from build123d import *

# Parameters (mm, degrees)
PAD005_DEPTH         = 2
POCKET003_DEPTH      = 2
SKETCH009_R          = 2.7
PAD004_DEPTH         = 5.9
SKETCH013_W          = 25
SKETCH013_H          = 50.4
SKETCH013_H_2        = 36.4
POCKET007_DEPTH      = 5.901
POCKET007_DEPTH_BACK = 0.001
SKETCH016_W          = 2.35
SKETCH016_H          = 50.4
PAD008_DEPTH         = 15
SKETCH017_W          = 2.35
SKETCH017_H          = 36.4
PAD009_DEPTH         = 5
SKETCH019_R          = 2.9
POCKET009_DEPTH      = 1.5
PAD011_DEPTH         = 5
SKETCH023_W          = 8
SKETCH023_H          = 4.5
SKETCH023_W_2        = 10
PAD013_DEPTH         = 7
SKETCH025_R          = 1.25
POCKET011_DEPTH      = 17.001
POCKET011_DEPTH_BACK = 0.001
SKETCH033_W          = 20
SKETCH033_H          = 50
POCKET017_DEPTH      = 17.001
POCKET017_DEPTH_BACK = 0.001
SKETCH042_W          = 15
SKETCH042_H          = 5.8
SKETCH042_H_2        = 3
POCKET021_DEPTH      = 17.001
POCKET021_DEPTH_BACK = 0.001


with BuildPart() as part:
    # Sketch011 → Pad005 (new body)
    with BuildSketch(Plane.XY):
        with BuildLine():
            Line((-29.5, -64), (29.5, -64))
            ThreePointArc((29.5, -64), (31.267767, -63.267767), (32, -61.5))
            Line((32, -42.5), (32, -61.5))
            ThreePointArc((34.5, -40), (32.732233, -40.732233), (32, -42.5))
            Line((34.5, 12), (34.5, -40))
            ThreePointArc((32, 14.5), (32.732233, 12.732233), (34.5, 12))
            Line((32, 21.5), (32, 14.5))
            ThreePointArc((32, 21.5), (31.267767, 23.267767), (29.5, 24))
            Line((29.5, 24), (-34.5, 24))
            ThreePointArc((-34.5, 24), (-36.267767, 23.267767), (-37, 21.5))
            Line((-37, 21.5), (-37, -40))
            ThreePointArc((-37, -40), (-36.267767, -41.767767), (-34.5, -42.5))
            ThreePointArc((-32, -45), (-32.732233, -43.232233), (-34.5, -42.5))
            Line((-32, -45), (-32, -61.5))
            ThreePointArc((-32, -61.5), (-31.267767, -63.267767), (-29.5, -64))
        make_face()
    extrude(amount=-PAD005_DEPTH)

    # Sketch007 → Pocket003 (cut)
    with BuildSketch(Plane.XY):
        Polygon((-21, 18.3), (-21, 5.3), (21, 5.3), (21, -3.7), (28, -3.7), (28, 18.3), align=None)
    extrude(amount=-POCKET003_DEPTH, mode=Mode.SUBTRACT)

    # Sketch009 → Pad004 (join)
    with BuildSketch(Plane.XY):
        with Locations((-18.25, -26)):
            Circle(SKETCH009_R)
        with Locations((12.75, -21)):
            Circle(SKETCH009_R)
        with Locations((18.25, 2.5027)):
            Circle(SKETCH009_R)
    extrude(amount=-PAD004_DEPTH)

    # Sketch013 → Pocket007 (cut, two sides)
    with BuildSketch(Plane.XY) as pocket007_sk:
        with Locations((-43.3, -8)):
            Rectangle(SKETCH013_W, SKETCH013_H)
        with Locations((43.3, -10)):
            Rectangle(SKETCH013_W, SKETCH013_H_2)
    extrude(amount=-POCKET007_DEPTH, mode=Mode.SUBTRACT)
    extrude(pocket007_sk.sketch, amount=POCKET007_DEPTH_BACK, mode=Mode.SUBTRACT)

    # Sketch016 (on Face5 of Pocket007) → Pad008 (join)
    with BuildSketch(Plane(origin=(0, 0, -2), x_dir=(1, 0, 0), z_dir=(0, 0, -1))):
        with Locations((-29.625, 8)):
            Rectangle(SKETCH016_W, SKETCH016_H)
    extrude(amount=PAD008_DEPTH)

    # Sketch017 (on Face5 of Pocket007) → Pad009 (join)
    with BuildSketch(Plane(origin=(0, 0, -2), x_dir=(1, 0, 0), z_dir=(0, 0, -1))):
        with Locations((29.625, 10)):
            Rectangle(SKETCH017_W, SKETCH017_H)
    extrude(amount=PAD009_DEPTH)

    # Sketch019 → Pocket009 (cut)
    with BuildSketch(Plane.XY):
        with Locations((-15, 21)):
            Circle(SKETCH019_R)
        with Locations((15, 21)):
            Circle(SKETCH019_R)
        with Locations((-15, -55)):
            Circle(SKETCH019_R)
        with Locations((15, -55)):
            Circle(SKETCH019_R)
    extrude(amount=-POCKET009_DEPTH, mode=Mode.SUBTRACT)

    # Sketch021 (on Face5 of Pocket009) → Pad011 (join)
    with BuildSketch(Plane(origin=(0, 0, -2), x_dir=(1, 0, 0), z_dir=(0, 0, -1))):
        with BuildLine():
            Line((-29.5, 64), (29.5, 64))
            ThreePointArc((32, 61.5), (31.267767, 63.267767), (29.5, 64))
            Line((32, 61.5), (32, 42.5))
            ThreePointArc((32, 42.5), (32.732233, 40.732233), (34.5, 40))
            Line((34.5, 28.2), (34.5, 40))
            Line((29, 28.2), (34.5, 28.2))
            Line((29, 58.5), (29, 28.2))
            Line((-29, 58.5), (29, 58.5))
            Line((-29, 39.5), (-29, 58.5))
            Line((-34, 39.5), (-29, 39.5))
            Line((-34, 33.2), (-34, 39.5))
            Line((-37, 33.2), (-34, 33.2))
            Line((-37, 40), (-37, 33.2))
            ThreePointArc((-34.5, 42.5), (-36.267767, 41.767767), (-37, 40))
            ThreePointArc((-34.5, 42.5), (-32.732233, 43.232233), (-32, 45))
            Line((-32, 61.5), (-32, 45))
            ThreePointArc((-29.5, 64), (-31.267767, 63.267767), (-32, 61.5))
        make_face()
        with BuildLine():
            Line((34.5, -8.2), (34.5, -12))
            ThreePointArc((34.5, -12), (32.732233, -12.732233), (32, -14.5))
            Line((32, -14.5), (32, -21.5))
            ThreePointArc((29.5, -24), (31.267767, -23.267767), (32, -21.5))
            Line((29.5, -24), (-34.5, -24))
            ThreePointArc((-37, -21.5), (-36.267767, -23.267767), (-34.5, -24))
            Line((-37, -21.5), (-37, -17.2))
            Line((-37, -17.2), (-36.26856, -17.2))
            Line((-36.26856, -17.2), (-36.26856, -18.5))
            Line((-36.26856, -18.5), (29, -18.5))
            Line((29, -18.5), (29, -8.2))
            Line((29, -8.2), (34.5, -8.2))
        make_face()
    extrude(amount=PAD011_DEPTH)

    # Sketch023 → Pad013 (join)
    with BuildSketch(Plane.XY):
        with Locations((-24, 20.45)):
            Rectangle(SKETCH023_W, SKETCH023_H)
        with Locations((25, 20.45)):
            Rectangle(SKETCH023_W, SKETCH023_H)
        with Locations((-18.5, -48.97)):
            Rectangle(SKETCH023_W_2, SKETCH023_H)
        with Locations((18.5, -48.97)):
            Rectangle(SKETCH023_W_2, SKETCH023_H)
    extrude(amount=-PAD013_DEPTH)

    # Sketch025 → Pocket011 (cut, two sides)
    with BuildSketch(Plane.XY) as pocket011_sk:
        with Locations((-34, 21)):
            Circle(SKETCH025_R)
        with Locations((27.5, 21)):
            Circle(SKETCH025_R)
        with Locations((27.5, -61)):
            Circle(SKETCH025_R)
        with Locations((-27.5, -61)):
            Circle(SKETCH025_R)
    extrude(amount=-POCKET011_DEPTH, mode=Mode.SUBTRACT)
    extrude(pocket011_sk.sketch, amount=POCKET011_DEPTH_BACK, mode=Mode.SUBTRACT)

    # Sketch033 → Pocket017 (cut, two sides)
    with BuildSketch(Plane.XY) as pocket017_sk:
        with Locations((0, -25)):
            Rectangle(SKETCH033_W, SKETCH033_H)
    extrude(amount=-POCKET017_DEPTH, mode=Mode.SUBTRACT)
    extrude(pocket017_sk.sketch, amount=POCKET017_DEPTH_BACK, mode=Mode.SUBTRACT)

    # Sketch042 → Pocket021 (cut, two sides)
    with BuildSketch(Plane.XY) as pocket021_sk:
        with Locations((-27.5, -35.7)):
            Rectangle(SKETCH042_W, SKETCH042_H)
        with Locations((25.7, -29.5)):
            Rectangle(SKETCH042_W, SKETCH042_H_2)
    extrude(amount=-POCKET021_DEPTH, mode=Mode.SUBTRACT)
    extrude(pocket021_sk.sketch, amount=POCKET021_DEPTH_BACK, mode=Mode.SUBTRACT)


solid = part.part
CAD build for the part. Positions are in the model's coordinates, mm. A direction names the side the tool comes from. Coordinates: 2 decimals unless noted, no trailing zeros. Write each loop counter-clockwise with the first axis right and the second up, starting at its lowest first coordinate (ties: lowest second). Pieces come first, ordered by that corner, then holes. Notation, with made-up numbers: M -21.75,61 L 20.25,61 A19 ccw 20.25,98 Z; hole C -33,81 d2. An arc over 180 degrees is marked long. Return JSON: item names as keys, results as strings.
Item 1: Drop flat-ended pins along their axis: pin 1 Ø7.5 at (y, z) = (16.5, -2.5) entering from +X; pin 2 Ø10 at (y, z) = (7.5, -9.5) entering from -X; pin 3 Ø10 at (y, z) = (-54, -6) entering from -X; pin 4 Ø2 at (x, y) = (27.5, 21) entering from +Z. Give the stop position or say it passes through.
Findings below:
{"pin 1": "stops at x = 32.71", "pin 2": "stops at x = -30.8", "pin 3": "stops at x = -32", "pin 4": "passes through"}
Item 2: Two-plate mould, pull along Y, no slides. Class faces 5 (the flat face through (32, -52, -3)), 6 (the flat face through (-15, -55, -1.5)), 7 (the flat face through (-2, 24, -3)): +Y half, -Y half, draft (parallel to the pull), parting line (faces both ways), or undercut.
Findings below:
{"face 5": "draft", "face 6": "undercut", "face 7": "+Y half"}
Item 3: Slice it at B-B, the plane x = -2. Write the cut outline in (y, z).
Findings below:
{"outline": "M -64,-7 L -58.5,-7 L -58.5,-2 L -50,-2 L -50,0 L -64,0 Z; M 0,-2 L 5.3,-2 L 5.3,0 L 0,0 Z; M 18.3,-2 L 18.5,-2 L 18.5,-7 L 24,-7 L 24,0 L 18.3,0 Z"}
Item 4: Slice it at D-D, the plane x = -19. Write the cut outline in (y, z), and give its area (3 significant figures).
Findings below:
{"outline": "M -64,-7 L -58.5,-7 L -58.5,-2 L -51.22,-2 L -51.22,-7 L -46.72,-7 L -46.72,-2 L -28.59,-2 L -28.59,-5.9 L -23.41,-5.9 L -23.41,-2 L 5.3,-2 L 5.3,0 L -64,0 Z; M 18.3,-2 L 18.5,-2 L 18.5,-7 L 24,-7 L 24,0 L 18.3,0 Z", "area": "248 mm2"}
Item 5: Slice it at A-A, the plane y = -36. Write the cut outline in (x, z), and give its area (4 significant figures).
Findings below:
{"outline": "M -37,-7 L -35,-7 L -35,0 L -37,0 Z; M -20,-2 L -10,-2 L -10,0 L -20,0 Z; M 10,-2 L 29,-2 L 29,-7 L 34.5,-7 L 34.5,0 L 10,0 Z", "area": "110.5 mm2"}
Item 6: Probe line 1 (X direction, y = 15.5, z = -4.5); line 2 (X direction, y = -51, z = -3); line 3 (Y direction, x = -12, z = -6). List the from-to ranges inside material, lowest first. Write a range as from..to.
Findings below:
{"line 1": "x = -30.8..-28.45, 29..32", "line 2": "x = -32..-29, -23.5..-13.5, 13.5..23.5, 29..32", "line 3": "y = -64..-58.5, 18.5..24"}
Item 7: Which spindle directions (+Z, -Z, +X, -X, +Y, -Y) get a long thin tool onto all of the face, cutting with end or side? Do faces 1 (the flat face through (30.8, -10, -3)), 2 (the flat face through (15, -55, -1.5)), 3 (the flat face through (29, -45, -4)), 4 (the flat face through (0, 0, -1)). Say none if no direction does.
Findings below:
{"face 1": "+Z, -Z, +X", "face 2": "+Z", "face 3": "-Z", "face 4": "+Z, -Z"}
Item 8: Slice it at C-C, the plane y = -9.5. Write the cut outline in (x, z), and give its area (3 significant figures).
Findings below:
{"outline": "M -30.8,-17 L -28.45,-17 L -28.45,-2 L -10,-2 L -10,0 L -30.8,0 Z; M 10,-2 L 28.45,-2 L 28.45,-7 L 30.8,-7 L 30.8,0 L 10,0 Z", "area": "130 mm2"}
